Build history of the part. All positions in model axes, mm. Give positions to 0.01 mm unless a question says otherwise; leave off trailing zeros. Loops run counter-clockwise (first coordinate to the right, second up) from the corner with the lowest first, then second, coordinate; pieces in that order, holes last. Notation, with made-up numbers: (55.5, -31) -> (102.5, -31) arc R19 ccw to (102.5, 6) -> close; hole circle Ø1 at (33.25, 5.5). An arc over 180 degrees is marked (long way). Answer as a JSON object with one key per item and string values. Group by question number.
Q1. Wall check: probe 1 along X at (y, z) = (16, 2.5); probe 2 along Y at (x, z) = (215, 1.5); probe 3 along Y at (x, z) = (254.5, 3). Give the ranges that are in metal, low to high. Write a range as from..to.
Q2. Band-saw the part on B-B, the plane x = 155.5. Write the cut outline in (y, z).
Q3. Drop a flat-ended pin along its axis: pin 1 (2.5 mm diameter, centred on x = 280, z = 2, fed in from +Y). Give the stop position or say it passes through.
Autodesk Inventor part; units mm, degrees
ref_plane "YZ Plane" through (0, 0, 0) normal (1, 0, 0) x (0, 1, 0)
ref_plane "XZ Plane" through (0, 0, 0) normal (0, 1, 0) x (-1, 0, 0)
ref_plane "XY Plane" through (0, 0, 0) normal (0, 0, 1) x (1, 0, 0)
sketch "Sketch1" plane through (0, 0, 0) normal (0, 0, 1) x (1, 0, 0)
  line L0 (0, 0) -> (430, 0)
  line L1 (430, 0) -> (430, 380)
  line L2 (430, 380) -> (0, 380)
  line L3 (0, 380) -> (0, 0)
  dimension "d0" = 430
  dimension "d1" = 380
extrude "Extrusion1" add sketch "Sketch1" along normal blind 4.7625
sketch "Sketch2" plane through (0, 0, 4.7625) normal (0, 0, 1) x (1, 0, 0)
  line L0 (0, 0) -> (430, 0)
  line L1 (430, 0) -> (430, 380)
  point P0 (215, 16)
  dimension "d8" = 215
  dimension "d33" = 16
hole "Hole1" at (215, 16, 4.7625) direction (0, 0, -1) diameter 3 end through all
sketch "Sketch4" plane through (0, 0, 4.7625) normal (0, 0, 1) x (1, 0, 0)
  line L0 (430, 380) -> (0, 380)
  line L1 (122.5, 380) -> (122.5, 372)
  line L2 (122.5, 372) -> (136.5, 372)
  line L3 (136.5, 372) -> (136.5, 360)
  line L4 (136.5, 360) -> (163.5, 360)
  line L5 (163.5, 360) -> (163.5, 372)
  line L6 (163.5, 372) -> (187.5, 372)
  line L7 (187.5, 372) -> (187.5, 334)
  line L8 (187.5, 334) -> (242.5, 334)
  line L9 (242.5, 334) -> (242.5, 372)
  line L10 (242.5, 372) -> (266.5, 372)
  line L11 (266.5, 372) -> (266.5, 360)
  line L12 (266.5, 360) -> (293.5, 360)
  line L13 (293.5, 360) -> (293.5, 372)
  line L14 (293.5, 372) -> (307.5, 372)
  line L15 (307.5, 372) -> (307.5, 380)
  point P0 (215, 380)
  point P1 (215, 334)
  dimension "d20" = 14
  dimension "d21" = 8
  dimension "d22" = 12
  dimension "d23" = 14
  dimension "d24" = 27
  dimension "d25" = 27
  dimension "d26" = 24
  dimension "d27" = 38
  dimension "d28" = 24
  dimension "d31" = 55
extrude "Extrusion2" cut sketch "Sketch4" against normal up to next
sketch "Sketch5" plane through (0, 0, 4.7625) normal (0, 0, 1) x (1, 0, 0)
  line L0 (122.5, 380) -> (0, 380)
  line L1 (0, 380) -> (0, 0)
  line L2 (430, 0) -> (430, 380)
  line L3 (430, 380) -> (307.5, 380)
  line L4 (94, 380) -> (94, 374)
  line L5 (94, 374) -> (102, 374)
  line L6 (102, 374) -> (102, 380)
  line L7 (327, 380) -> (327, 374)
  line L8 (327, 374) -> (335, 374)
  line L9 (335, 374) -> (335, 380)
  dimension "d36" = 8
  dimension "d37" = 94
  dimension "d38" = 6
  dimension "d39" = 95
extrude "Extrusion3" cut sketch "Sketch5" against normal up to next
sketch "Sketch6" plane through (0, 0, 4.7625) normal (0, 0, 1) x (1, 0, 0)
  line L0 (102, 380) -> (102, 374)
  line L1 (122.5, 380) -> (102, 380)
  line L2 (108, 380) -> (112, 380)
  line L3 (112, 380) -> (112, 377)
  line L4 (112, 377) -> (108, 377)
  line L5 (108, 377) -> (108, 380)
  dimension "d46" = 4
  dimension "d47" = 3
  dimension "d48" = 6
extrude "Extrusion4" cut sketch "Sketch6" against normal up to next
properties part number "ElectronicsTopPanel" material "ABS Plastic"
Worked answers:
{
 "1": {"probe 1": "0..213.5, 216.5..430", "probe 2": "0..14.5, 17.5..334", "probe 3": "0..372"},
 "2": {"outline": "(0, 0) -> (360, 0) -> (360, 4.76) -> (0, 4.76) -> close"},
 "3": {"pin 1": "y = 360"}
}
